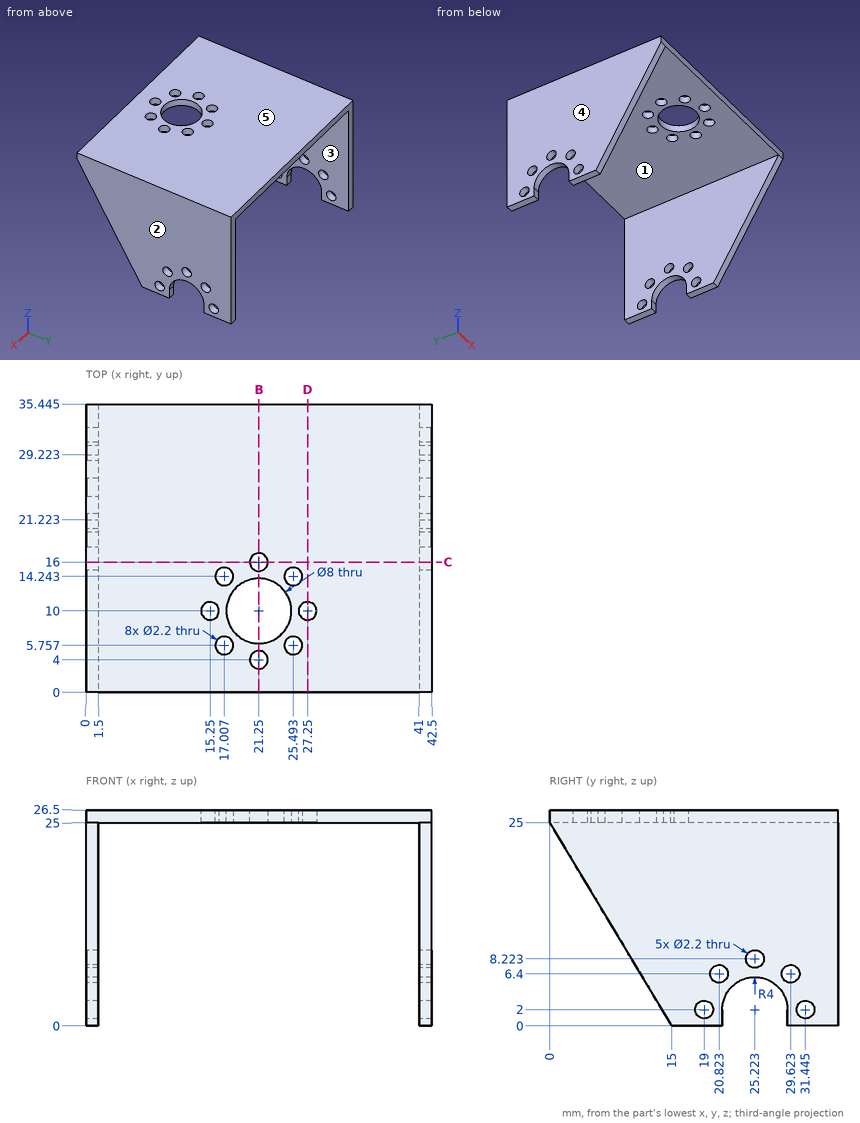
Geometry check sheet. Reference: drawing and pictorial views, mm from the part's lowest x, y, z. A direction names the side the tool comes from. Round coordinates to 2 decimals unless told otherwise and drop trailing zeros. Loops run counter-clockwise (first coordinate to the right, second up) from the corner with the lowest first, then second, coordinate; pieces in that order, holes last. Notation, with made-up numbers: (42, -27) -> (50, -27) arc R23 ccw to (50, 5) -> close; hole circle Ø3 at (-29, 27.25). An arc over 180 degrees is marked (long way). Answer as a JSON object with one key per item and string values. Group by question number.
Item 1: Depth check by flat-ended pin: pin 1 Ø3 at (x, y) = (15.25, 10) entering from -Z; pin 2 Ø1.8 at (x, y) = (25.49, 14.24) entering from -Z; pin 3 Ø1.2 at (x, z) = (42, 0.5) entering from -Y. Enter the tip coordinate at first touch or a pass-through.
Item 2: Thickness scan on line 1 along Y through (x, z) = (21.25, 25.9) (1 decimal); line 2 along X through (y, z) = (19.5, 16.75); line 3 along Z through (x, y) = (3, 14.5). Record the ranges inside material, lowest first.
Item 3: Release check for a two-part mould opening along X. For the marked faces 3, 4 and 5 record: pulls with the +X half, pulls with the -X half, needs draft (parallel to the pull), parting line crosses it, or undercut.
Item 4: Cross-section at C-C, the plane y = 16. Record the cut outline in (x, z).
Item 5: Set-up check for the marked faces 1 and 2: record each of +Z, -Z, +X, -X, +Y, -Y from which the full face is reachable in a straight line by a thin tool's end or side.
Item 6: Cross-section at D-D, the plane x = 27.25. Record the cut outline in (y, z) (1 decimal).
Item 7: Cross-section at B-B, the plane x = 21.25. Record the cut outline in (y, z) (1 decimal).
Determined:
{
 "1": {"pin 1": "stops at z = 25", "pin 2": "passes through", "pin 3": "stops at y = 14.34"},
 "2": {"line 1": "y = 0 to 2.9, 5.1 to 6, 14 to 14.9, 17.1 to 35.4", "line 2": "x = 0 to 1.5, 41 to 42.5", "line 3": "z = 25 to 26.5"},
 "3": {"face 3": "undercut", "face 4": "pulls with the -X half", "face 5": "needs draft"},
 "4": {"outline": "(0, 0) -> (1.5, 0) -> (1.5, 25) -> (20.15, 25) -> (20.15, 26.5) -> (0, 26.5) -> close; (22.35, 25) -> (41, 25) -> (41, 0) -> (42.5, 0) -> (42.5, 26.5) -> (22.35, 26.5) -> close"},
 "5": {"face 1": "-Z, +Y, -Y", "face 2": "+Z, -Z, +X, +Y, -Y"},
 "6": {"outline": "(0, 25) -> (8.9, 25) -> (8.9, 26.5) -> (0, 26.5) -> close; (11.1, 25) -> (35.4, 25) -> (35.4, 26.5) -> (11.1, 26.5) -> close"},
 "7": {"outline": "(0, 25) -> (2.9, 25) -> (2.9, 26.5) -> (0, 26.5) -> close; (5.1, 25) -> (6, 25) -> (6, 26.5) -> (5.1, 26.5) -> close; (14, 25) -> (14.9, 25) -> (14.9, 26.5) -> (14, 26.5) -> close; (17.1, 25) -> (35.4, 25) -> (35.4, 26.5) -> (17.1, 26.5) -> close"}
}
